Work out the finished part from the listing and answer in its coordinate system (mm). Face numbers are marked on the shaded views. A direction names the side the tool comes from. Round coordinates to 2 decimals unless told otherwise and drop trailing zeros. Loops run counter-clockwise (first coordinate to the right, second up) from the corner with the lowest first, then second, coordinate; pieces in that order, holes last. Notation, with made-up numbers: M -12,13.25 L 32,13.25 A21 cw 32,18.25 Z; hole C 44,45 d5. An arc over 180 degrees is marked long. One line per item, written item: value.
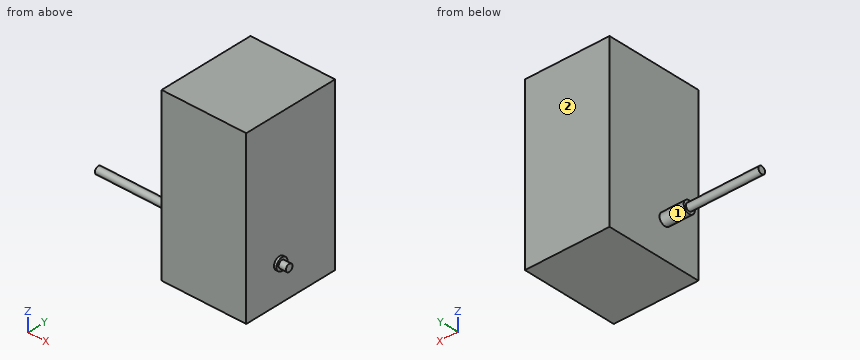
Autodesk Inventor part; units mm, degrees
ref_plane "YZ Plane" through (0, 0, 0) normal (1, 0, 0) x (0, 1, 0)
ref_plane "XZ Plane" through (0, 0, 0) normal (0, 1, 0) x (-1, 0, 0)
ref_plane "XY Plane" through (0, 0, 0) normal (0, 0, 1) x (1, 0, 0)
sketch "Skizze1" plane through (0, 0, 0) normal (0, 1, 0) x (-1, 0, 0)
  line L0 (52.027, -65.0338) -> (17.027, -65.0338)
  line L1 (17.027, -65.0338) -> (17.027, -135.0338)
  line L2 (17.027, -135.0338) -> (52.027, -135.0338)
  line L3 (52.027, -135.0338) -> (52.027, -65.0338)
  point P0 (0, 0)
  dimension "d0" = 70
  dimension "d1" = 35
extrude "Extrusion1" add sketch "Skizze1" along normal blind 40
sketch "Skizze2" plane through (-17.027, 0, -65.0338) normal (1, 0, 0) x (0, 0, -1)
  circle A0 centre (55, 15) radius 1.5
  circle A1 centre (55, 15) radius 2.5
  line L0 (0, 0) -> (70, 0)
  line L1 (70, 0) -> (70, 40)
  point P0 (-65.0338, 0)
  dimension "d4" = 3
  dimension "d5" = 5
  dimension "d6" = 15
  dimension "d7" = 15
extrude "Extrusion2" add sketch "Skizze2" along normal blind 4 contours A0
extrude "Extrusion3" add sketch "Skizze2" along normal blind 1
sketch "Skizze3" plane through (-52.027, 0, -135.0338) normal (-1, 0, 0) x (0, 0, 1)
  circle A0 centre (15, 15) radius 1.5
  circle A1 centre (15, 15) radius 2.5
  line L0 (0, 0) -> (0, 40)
  line L1 (0, 0) -> (70, 0)
  point P0 (-65.0338, 0)
  dimension "d12" = 3
  dimension "d13" = 5
  dimension "d16" = 15
  dimension "d17" = 15
extrude "Extrusion4" add sketch "Skizze3" along normal blind 40 contours A0
extrude "Extrusion5" add sketch "Skizze3" along normal blind 10
properties part number "Motor_links"
1) Each of these flat-tipped pins is pushed along its axis until it touches: pin 1 (5 mm diameter, centred on x = -53.5, z = -74, fed in from +Y); pin 2 (8 mm diameter, centred on x = -70.5, z = -112, fed in from +Y); pin 3 (1 mm diameter, centred on y = 17.5, z = -110.5, fed in from -X); pin 4 (12 mm diameter, centred on y = 30, z = -127, fed in from +X). Where does it stop, or does it pass through?
Check values:
pin 1: y = 40
pin 2: through
pin 3: x = -52.03
pin 4: x = -17.03
2) Find section D-D (y = 29). Give the vertices of the cut face in (x, z).
Check values:
outline: M -52.03,-135.03 L -17.03,-135.03 L -17.03,-65.03 L -52.03,-65.03 Z
3) Find section B-B (z = -116). Give the vertices of the cut face in (x, y).
Check values:
outline: M -52.03,0 L -17.03,0 L -17.03,40 L -52.03,40 Z
4) For the marked faces 1 and 2, determine the directions among +Z, -Z, +X, -X, +Y, -Y from which every point of the face is accessible in a straight line to the end or side of a thin tool.
Check values:
face 1: -X
face 2: +Z, -Z, +X, -X, +Y
5) Find section A-A (y = 15). Give the vertices of the cut face in (x, z).
Check values:
outline: M -92.03,-121.53 L -62.03,-121.53 L -62.03,-122.53 L -52.03,-122.53 L -52.03,-135.03 L -17.03,-135.03 L -17.03,-122.53 L -16.03,-122.53 L -16.03,-121.53 L -13.03,-121.53 L -13.03,-118.53 L -16.03,-118.53 L -16.03,-117.53 L -17.03,-117.53 L -17.03,-65.03 L -52.03,-65.03 L -52.03,-117.53 L -62.03,-117.53 L -62.03,-118.53 L -92.03,-118.53 Z
6) Find the intervals of material crossed by probe 1 along X at (y, z) = (6, -113); probe 2 along Y at (x, z) = (-74, -119); probe 3 along Z at (x, y) = (-70.5, 14), in increasing order. Write a range as from..to.
Check values:
probe 1: -52.03..-17.03
probe 2: 13.91..16.09
probe 3: -121.15..-118.92
7) Find section C-C (x = -78). Give the vertices of the cut face in (y, z).
Check values:
outline: C 15,-120.03 d3
